Source: CAD feature listing. Evaluate the final solid. Frame: model axes, mm. Round coordinates to 2 decimals unless told otherwise and drop trailing zeros. Loops run counter-clockwise (first coordinate to the right, second up) from the corner with the lowest first, then second, coordinate; pieces in that order, holes last. Notation, with made-up numbers: (-16, -26) - (32, -26) arc R18 cw to (32, 9) - close; hole circle Ø3 at (3, 10). An arc over 180 degrees is marked (long way). One line per question, with ' | ' between items. Start each with the question number.
1. Cut plane B-B (x = 23.5). Return loops of the section in (y, z).
2. Cut plane C-C (z = 1.75). Return loops of the section in (x, y), then the cut area to 3 significant figures.
3. Ray query, line 1 (Y direction, x = 0, z = 3.55); line 2 (Y direction, x = 25.5, z = 2.45); line 3 (X direction, y = 54, z = 0.4). Return the intervals inside material, ascending.
4. Cut plane A-A (y = -65). Return loops of the section in (x, z).
```python
from build123d import *

# Parameters (mm, degrees)
ESQUISSE1_W              = 120
ESQUISSE1_H              = 832
BOSS_EXTRU_1_DEPTH       = 6
CUT_EXTRUDE1_DEPTH       = 10
M6_CLEARANCE_HOLE1_D     = 6.6
M6_CLEARANCE_HOLE1_DEPTH = 6
M6_CLEARANCE_HOLE1_TIP   = 1.982840043


with BuildPart() as part:
    # Esquisse1 → Boss.-Extru.1 (new body)
    with BuildSketch(Plane.XY):
        Rectangle(ESQUISSE1_W, ESQUISSE1_H)
    extrude(amount=BOSS_EXTRU_1_DEPTH)

    # Sketch1 → Cut-Extrude1 (cut)
    with BuildSketch(Plane.XY.offset(6)):
        with BuildLine():
            Line((-42, 376.726304266), (-42, -233.273695734))
            ThreePointArc((-42, -233.273695734), (-39.071067812, -240.344763545), (-32, -243.273695734))
            Line((-32, -243.273695734), (32, -243.273695734))
            ThreePointArc((32, -243.273695734), (39.071067812, -240.344763545), (42, -233.273695734))
            Line((42, -233.273695734), (42, 376.726304266))
            ThreePointArc((42, 376.726304266), (39.071067812, 383.797372078), (32, 386.726304266))
            Line((32, 386.726304266), (-32, 386.726304266))
            ThreePointArc((-32, 386.726304266), (-39.071067812, 383.797372078), (-42, 376.726304266))
        make_face()
    extrude(amount=-CUT_EXTRUDE1_DEPTH, mode=Mode.SUBTRACT)

    # M6 Clearance Hole1
    with Locations(Plane.XY.offset(6)):
        with Locations((0, 390.726304266), (0, -247.273695734)):
            Hole(M6_CLEARANCE_HOLE1_D / 2, depth=M6_CLEARANCE_HOLE1_DEPTH)
            with Locations((0, 0, -(M6_CLEARANCE_HOLE1_DEPTH + M6_CLEARANCE_HOLE1_TIP / 2))):  # 118° drill point
                Cone(0, M6_CLEARANCE_HOLE1_D / 2, M6_CLEARANCE_HOLE1_TIP, mode=Mode.SUBTRACT)


solid = part.part
```
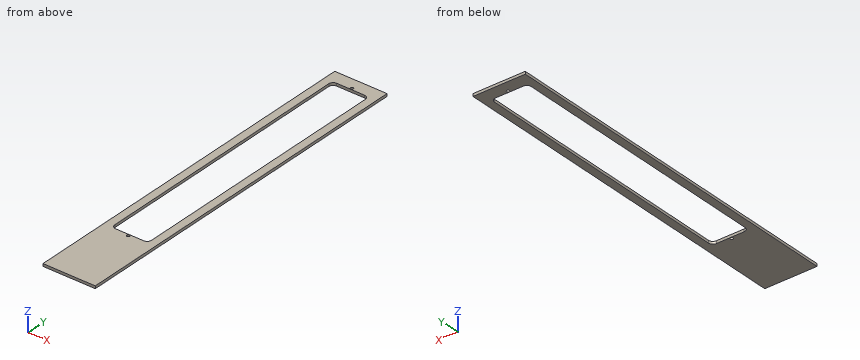
Answers follow:
1) outline: (-416, 0) - (-243.27, 0) - (-243.27, 6) - (-416, 6) - close; (386.73, 0) - (416, 0) - (416, 6) - (386.73, 6) - close
2) outline: (-60, -416) - (60, -416) - (60, 416) - (-60, 416) - close; hole (-42, -233.27) arc R10 ccw to (-32, -243.27) - (32, -243.27) arc R10 ccw to (42, -233.27) - (42, 376.73) arc R10 ccw to (32, 386.73) - (-32, 386.73) arc R10 ccw to (-42, 376.73) - close; hole circle Ø6.6 at (0, -247.27); hole circle Ø6.6 at (0, 390.73) | area: 46,900 mm2
3) line 1: y = -416 to -250.57, -243.97 to -243.27, 386.73 to 387.43, 394.03 to 416 | line 2: y = -416 to -243.27, 386.73 to 416 | line 3: x = -60 to -42, 42 to 60
4) outline: (-60, 0) - (-42, 0) - (-42, 6) - (-60, 6) - close; (42, 0) - (60, 0) - (60, 6) - (42, 6) - close
